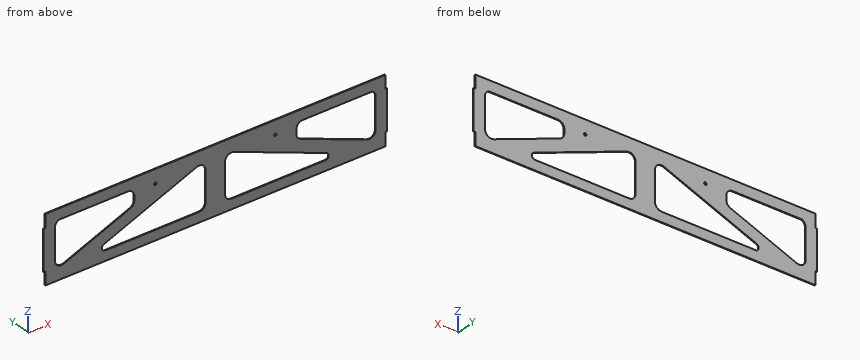
from build123d import *

# Parameters (mm, degrees)
BOSS_EXTRUDE1_DEPTH = 1.5875
CUT_EXTRUDE2_DEPTH  = 343.657797193
SKETCH4_R           = 2.5
CUT_EXTRUDE3_DEPTH  = 343.657797193


with BuildPart() as part:
    # Sketch1 → Boss-Extrude1 (new body)
    with BuildSketch(Plane(origin=(0, 0, 0), x_dir=(1, 0, 0), z_dir=(0, 1, 0))):
        Polygon((-333.375, 38.989), (-333.375, 64.389), (333.375, 64.389), (333.375, 38.989), (336.55, 38.989), (336.55, -38.989), (333.375, -38.989), (333.375, -64.389), (-333.375, -64.389), (-333.375, -38.989), (-336.55, -38.989), (-336.55, 38.989), align=None)
    extrude(amount=BOSS_EXTRUDE1_DEPTH)

    # Sketch3 → Cut-Extrude2 (cut, through all)
    with BuildSketch(Plane(origin=(0, 1.5875, 0), x_dir=(1, 0, 0), z_dir=(0, 1, 0))):
        with BuildLine():
            Line((-314.325, 26.808799864), (-314.325, -32.639))
            ThreePointArc((-314.325, -32.639), (-312.428265266, -39.315785124), (-307.304612663, -43.998225326))
            Line((-307.304612663, -43.998225326), (-171.45, -43.998225326))
            ThreePointArc((-171.45, -43.998225326), (-162.469743879, -40.278481447), (-158.75, -31.298225326))
            Line((-158.75, -31.298225326), (-158.75, -23.549607936))
            ThreePointArc((-158.75, -23.549607936), (-160.974250295, -16.369867821), (-166.867900491, -11.705015748))
            Line((-166.867900491, -11.705015748), (-297.042900491, 38.653392051))
            ThreePointArc((-297.042900491, 38.653392051), (-308.804740115, 37.284549569), (-314.325, 26.808799864))
        make_face()
        with BuildLine():
            Line((-215.969521054, 45.339), (-31.75, 45.339))
            ThreePointArc((-31.75, 45.339), (-22.769743879, 41.619256121), (-19.05, 32.639))
            Line((-19.05, 32.639), (-19.05, -25.46802519))
            ThreePointArc((-19.05, -25.46802519), (-24.570259885, -35.943774895), (-36.332099509, -37.312617377))
            Line((-36.332099509, -37.312617377), (-218.260570808, 33.066703906))
            ThreePointArc((-218.260570808, 33.066703906), (-222.211679342, 40.154315366), (-215.969521054, 45.339))
        make_face()
        with BuildLine():
            Line((36.332099509, -37.312617377), (218.260570808, 33.066703906))
            ThreePointArc((218.260570808, 33.066703906), (222.211679342, 40.154315366), (215.969521054, 45.339))
            Line((215.969521054, 45.339), (31.75, 45.339))
            ThreePointArc((31.75, 45.339), (22.769743879, 41.619256121), (19.05, 32.639))
            Line((19.05, 32.639), (19.05, -25.46802519))
            ThreePointArc((19.05, -25.46802519), (24.570259885, -35.943774895), (36.332099509, -37.312617377))
        make_face()
        with BuildLine():
            Line((314.325, 26.808799864), (314.325, -32.639))
            ThreePointArc((314.325, -32.639), (312.428265266, -39.315785124), (307.304612663, -43.998225326))
            Line((307.304612663, -43.998225326), (171.45, -43.998225326))
            ThreePointArc((171.45, -43.998225326), (162.469743879, -40.278481447), (158.75, -31.298225326))
            Line((158.75, -31.298225326), (158.75, -23.549607936))
            ThreePointArc((158.75, -23.549607936), (160.974250295, -16.369867821), (166.867900491, -11.705015748))
            Line((166.867900491, -11.705015748), (297.042900491, 38.653392051))
            ThreePointArc((297.042900491, 38.653392051), (308.804740115, 37.284549569), (314.325, 26.808799864))
        make_face()
    extrude(amount=-CUT_EXTRUDE2_DEPTH, mode=Mode.SUBTRACT)

    # Sketch4 → Cut-Extrude3 (cut, through all)
    with BuildSketch(Plane(origin=(0, 1.5875, 0), x_dir=(1, 0, 0), z_dir=(0, 1, 0))):
        with Locations(Location((-117.729, -37.465, 0), (0, 0, 270))):
            Circle(SKETCH4_R)
        with Locations(Location((117.729, -37.465, 0), (0, 0, 90))):
            Circle(SKETCH4_R)
    extrude(amount=-CUT_EXTRUDE3_DEPTH, mode=Mode.SUBTRACT)


solid = part.part
Model file for the job. Use its own axes, mm. Round coordinates to 2 decimals unless told otherwise and drop trailing zeros. Order: outer loops, then holes, each group sorted by start corner. A loop starts at its lowest first (then second) coordinate and runs counter-clockwise, first axis right, second up.
(1) Band-saw the part on C-C (x = -272). List the corners of the cut face in (y, z).
(2) Band-saw the part on B-B (x = -42). List the corners of the cut face in (y, z).
(3) Drill centre lines: line 1 (Z direction, x = -298, y = 1); line 2 (Z direction, x = 186, y = 1.4); line 3 (X direction, y = 0.65, z = -52) (3 decimals). Where is each one in solid material? Low to high.
(4) Pin check, flat tips, straight feed: pin 1 (8 mm diameter, centred on x = 108.5, z = 43.5, fed in from -Y); pin 2 (0.5 mm diameter, centred on y = 0.5, z = 49, fed in from -X) (3 decimals); pin 3 (0.8 mm diameter, centred on x = 335.5, y = 0.5, fed in from -Z); pin 4 (0.8 mm diameter, centred on y = 0.5, z = -49.5, fed in from +X) (3 decimals). Stop position of each tip, or through.
(5) Band-saw the part on A-A (z = -2). Give the number of separate pieces and of enclosed holes in the cut face, then the cut area to 3 significant figures.
Verdict:
1. outline: (0, -64.39) - (1.59, -64.39) - (1.59, -28.97) - (0, -28.97) - close; (0, 44) - (1.59, 44) - (1.59, 64.39) - (0, 64.39) - close
2. outline: (0, -64.39) - (1.59, -64.39) - (1.59, -45.34) - (0, -45.34) - close; (0, 35.12) - (1.59, 35.12) - (1.59, 64.39) - (0, 64.39) - close
3. line 1: z = -64.39 to -38.98, 44 to 64.39
3. line 2: z = -64.39 to -45.34, -20.59 to 4.3, 44 to 64.39
3. line 3: x = -333.375 to 333.375
4. pin 1: stops at y = 0
4. pin 2: stops at x = -333.375
4. pin 3: stops at z = -38.99
4. pin 4: stops at x = 333.375
5. separate pieces: 5
5. enclosed holes: 0
5. area: 335 mm2
